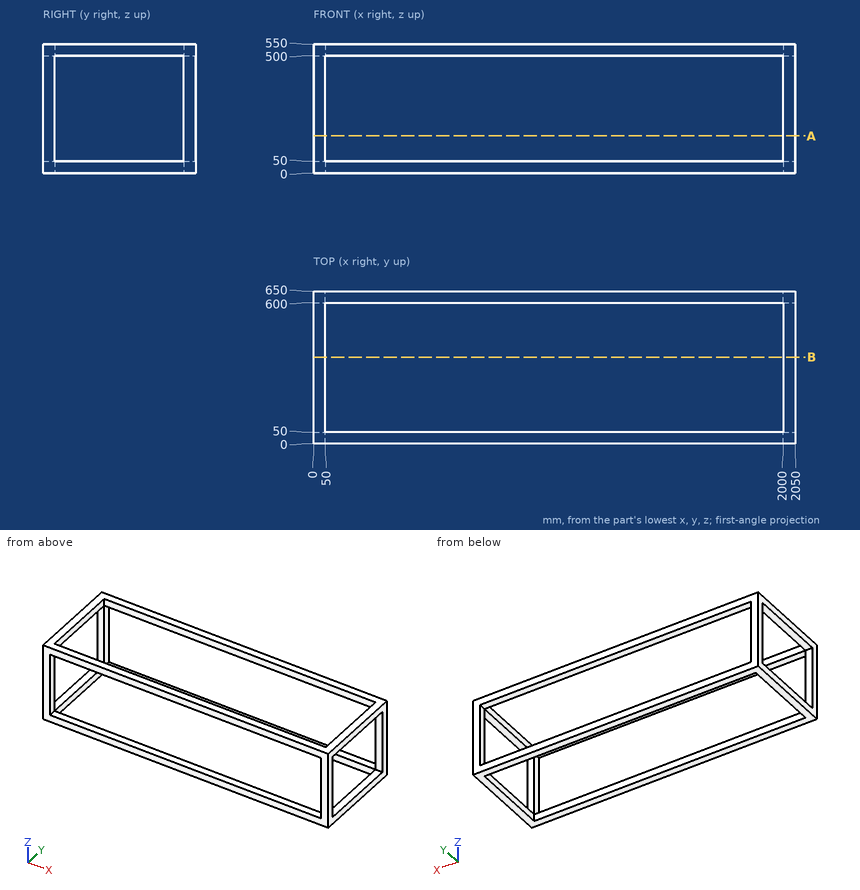
Print and shaded views of the part. All mm, measured from the part's lowest x, y and z. Round coordinates to 2 decimals unless told otherwise and drop trailing zeros. Write each loop counter-clockwise with the first axis right and the second up, starting at its lowest first coordinate (ties: lowest second). Pieces come first, ordered by that corner, then holes. Notation, with made-up numbers: (79.5, 29.5) - (94.5, 29.5) arc R16 cw to (94.5, 53.5) - close; hole circle Ø8 at (18, 63.25). An arc over 180 degrees is marked (long way). Write each question's results on one line, items separated by ' | '. Start each with the question number.
Item 1: Saw through at B-B (y = 369.5). Write the cut outline in (x, z), and give its area (3 significant figures).
Item 2: Wall check: L1, parallel to X at y = 454, z = 506; L2, parallel to Z at x = 167.5, y = 27.5; L3, parallel to Y at x = 494, z = 503. Give the ranges that are in metal, low to high. Write a range as [from, to].
Item 3: Saw through at A-A (z = 158.5). Write the cut outline in (x, y).
Results are:
1) outline: (0, 0) - (50, 0) - (50, 50) - (0, 50) - close; (0, 500) - (50, 500) - (50, 550) - (0, 550) - close; (2000, 0) - (2050, 0) - (2050, 50) - (2000, 50) - close; (2000, 500) - (2050, 500) - (2050, 550) - (2000, 550) - close | area: 10,000 mm²
2) L1: x = [0, 50], [2000, 2050] | L2: z = [0, 50], [500, 550] | L3: y = [0, 50], [600, 650]
3) outline: (0, 0) - (50, 0) - (50, 50) - (0, 50) - close; (0, 600) - (50, 600) - (50, 650) - (0, 650) - close; (2000, 0) - (2050, 0) - (2050, 50) - (2000, 50) - close; (2000, 600) - (2050, 600) - (2050, 650) - (2000, 650) - close
